Can you work these out from the drawing? Everything is in mm from the part's minimum corner. A direction names the side the tool comes from. Coordinates: 2 decimals unless noted, no trailing zeros. Order: outer loops, then holes, each group sorted by start corner. A loop starts at its lowest first (then second) coordinate and runs counter-clockwise, first axis right, second up. Notation, with made-up numbers: (-35.5, 31) -> (2.5, 31) arc R27 ccw to (2.5, 70) -> close; hole circle Ø8 at (-5, 82.25). An arc over 180 degrees is marked (long way). Put each result on its own line as item: value. Start each with the question number.
Q1. For the marked faces 1, 2 and 3, which set-ups out of +Z, -Z, +X, -X, +Y, -Y let a thin tool reach every point of the face, with its end or its side?
Q2. If we section it at B-B (y = 5.5): Please give me the cut outline in (x, z).
Q3. Will these pins go through, and if not, where does the flat tip stop? pin 1 (8 mm diameter, centred on x = 1.5, z = 36, fed in from -Y); pin 2 (8 mm diameter, centred on y = 4, z = 10.5, fed in from +X); pin 3 (2 mm diameter, centred on x = 2, y = 5, fed in from +Z).
Q4. If we section it at C-C (z = 25.5): Please give me the cut outline in (x, y).
Q5. If we section it at A-A (x = 7): Please give me the cut outline in (y, z), and give its area (3 significant figures).
Q6. If we section it at D-D (y = 14.75): Please give me the cut outline in (x, z), and give its area (3 significant figures).
Q7. Please list where these lines run through material, in increasing order: line 1 along Z through (x, y) = (4.25, 3); line 2 along Y through (x, z) = (6.75, 8) (1 decimal); line 3 along Z through (x, y) = (9.25, 4.75).
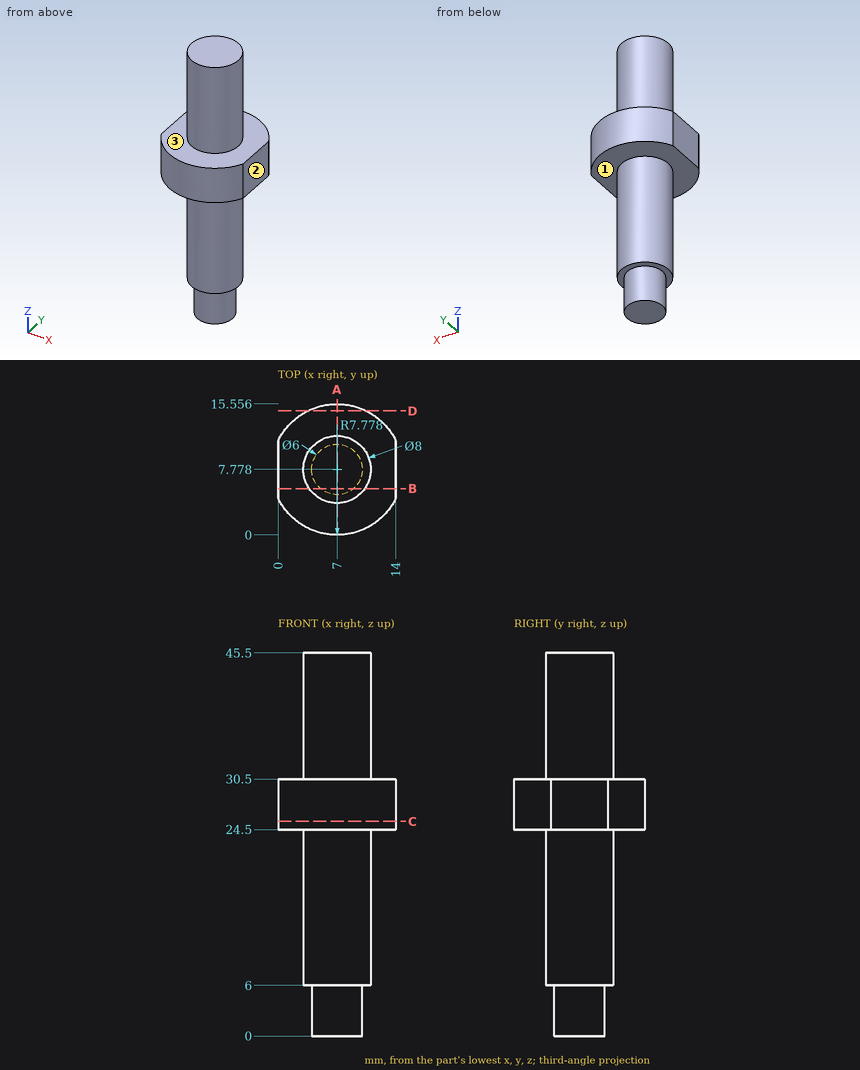
The answers:
1. face 1: -Z
1. face 2: +Z, -Z, +X, +Y, -Y
1. face 3: +Z
2. outline: (0, 24.5) -> (3.71, 24.5) -> (3.71, 6) -> (5.05, 6) -> (5.05, 0) -> (8.95, 0) -> (8.95, 6) -> (10.29, 6) -> (10.29, 24.5) -> (14, 24.5) -> (14, 30.5) -> (10.29, 30.5) -> (10.29, 45.5) -> (3.71, 45.5) -> (3.71, 30.5) -> (0, 30.5) -> close
3. pin 1: y = 4.07
3. pin 2: x = 11
3. pin 3: z = 30.5
4. outline: (0, 4.39) arc R7.78 ccw to (14, 4.39) -> (14, 11.17) arc R7.78 ccw to (0, 11.17) -> close
5. outline: (0, 24.5) -> (3.78, 24.5) -> (3.78, 6) -> (4.78, 6) -> (4.78, 0) -> (10.78, 0) -> (10.78, 6) -> (11.78, 6) -> (11.78, 24.5) -> (15.56, 24.5) -> (15.56, 30.5) -> (11.78, 30.5) -> (11.78, 45.5) -> (3.78, 45.5) -> (3.78, 30.5) -> (0, 30.5) -> close
5. area: 397 mm^2
6. outline: (3.55, 24.5) -> (10.45, 24.5) -> (10.45, 30.5) -> (3.55, 30.5) -> close
6. area: 41.4 mm^2
7. line 1: 24.5 to 30.5
7. line 2: 3.8 to 11.8
7. line 3: 6 to 45.5
